Here's how the part is built. I have some questions about the finished solid (model axes, mm). Coordinates: 2 decimals unless noted, no trailing zeros. Write each loop counter-clockwise with the first axis right and the second up, starting at its lowest first coordinate (ties: lowest second). Pieces come first, ordered by that corner, then holes.
Item 1: If we section it at C-C (z = 3.4): Count the separate pieces of the cut face and the enclosed holes in it, then the cut area to 3 significant figures.
Item 2: If we section it at B-B (x = 390.5): Please give me the cut outline in (y, z).
Item 3: If I drill on line 1 (X direction, y = 30, z = 3.5); line 2 (Y direction, x = 30, z = 2.1); line 3 (Y direction, x = 403, z = 1.2), over which ranges is the centre line in solid material (lowest first)?
Item 4: If we section it at A-A (x = 97.5): Please give me the cut outline in (y, z), then the cut area to 3 significant figures.
from build123d import *

# Parameters (mm, degrees)
BOSS_EXTRU_1_DEPTH         = 5
D_GAGEMENT_M51_D           = 5.5
D_GAGEMENT_M51_CSINK_D     = 5.55
D_GAGEMENT_M51_CSINK_ANGLE = 90
ENL_V_MAT_EXTRU_1_DEPTH    = 560.039354608
D_GAGEMENT_M52_D           = 5.5
D_GAGEMENT_M52_CSINK_D     = 6
D_GAGEMENT_M52_CSINK_ANGLE = 90
ENL_V_MAT_EXTRU_2_DEPTH    = 560.039354608
ENL_V_MAT_EXTRU_3_DEPTH    = 560.039354608
ESQUISSE15_R               = 2.5
ENL_V_MAT_EXTRU_4_DEPTH    = 560.039354608


with BuildPart() as part:
    # Esquisse1 → Boss.-Extru.1 (new body)
    with BuildSketch(Plane.XY):
        with BuildLine():
            Line((30, 0), (470, 0))
            ThreePointArc((470, 0), (491.213203436, 8.786796564), (500, 30))
            Line((500, 30), (500, 220))
            ThreePointArc((500, 220), (491.213203436, 241.213203436), (470, 250))
            Line((470, 250), (30, 250))
            ThreePointArc((30, 250), (8.786796564, 241.213203436), (0, 220))
            Line((0, 220), (0, 30))
            ThreePointArc((0, 30), (8.786796564, 8.786796564), (30, 0))
        make_face()
    extrude(amount=BOSS_EXTRU_1_DEPTH)

    # Dégagement M51 (through all)
    with Locations(Plane(origin=(0, 0, 0), x_dir=(-1, 0, 0), z_dir=(0, 0, -1))):
        with Locations((-470, 220), (-470, 30), (-30, 30), (-30, 220)):
            CounterSinkHole(D_GAGEMENT_M51_D / 2, D_GAGEMENT_M51_CSINK_D / 2, counter_sink_angle=D_GAGEMENT_M51_CSINK_ANGLE)

    # Esquisse8 → Enlèv. mat.-Extru.1 (cut, through all)
    with BuildSketch(Plane.XY.offset(5)):
        with BuildLine():
            Line((72, 225), (152, 225))
            ThreePointArc((152, 225), (153.414213562, 224.414213562), (154, 223))
            Line((154, 223), (154, 215))
            ThreePointArc((154, 215), (153.414213562, 213.585786438), (152, 213))
            Line((152, 213), (72, 213))
            ThreePointArc((72, 213), (70.585786438, 213.585786438), (70, 215))
            Line((70, 215), (70, 223))
            ThreePointArc((70, 223), (70.585786438, 224.414213562), (72, 225))
        make_face()
        with BuildLine():
            Line((346, 223), (346, 215))
            ThreePointArc((346, 215), (346.585786438, 213.585786438), (348, 213))
            Line((348, 213), (428, 213))
            ThreePointArc((428, 213), (429.414213562, 213.585786438), (430, 215))
            Line((430, 215), (430, 223))
            ThreePointArc((430, 223), (429.414213562, 224.414213562), (428, 225))
            Line((428, 225), (348, 225))
            ThreePointArc((348, 225), (346.585786438, 224.414213562), (346, 223))
        make_face()
    extrude(amount=-ENL_V_MAT_EXTRU_1_DEPTH, mode=Mode.SUBTRACT)

    # Dégagement M52 (through all)
    with Locations(Plane.XY.offset(5)):
        with Locations((60, 238), (440, 238), (250, 238)):
            CounterSinkHole(D_GAGEMENT_M52_D / 2, D_GAGEMENT_M52_CSINK_D / 2, counter_sink_angle=D_GAGEMENT_M52_CSINK_ANGLE)

    # Esquisse13 → Enlèv. mat.-Extru.2 (cut, through all)
    with BuildSketch(Plane(origin=(0, 0, 0), x_dir=(-1, 0, 0), z_dir=(0, 0, -1))):
        with BuildLine():
            Line((-105, 88), (-105, 62))
            ThreePointArc((-105, 62), (-104.414213562, 60.585786438), (-103, 60))
            Line((-103, 60), (-82, 60))
            ThreePointArc((-82, 60), (-80.585786438, 60.585786438), (-80, 62))
            Line((-80, 62), (-80, 88))
            ThreePointArc((-80, 88), (-80.585786438, 89.414213562), (-82, 90))
            Line((-82, 90), (-103, 90))
            ThreePointArc((-103, 90), (-104.414213562, 89.414213562), (-105, 88))
        make_face()
    extrude(amount=-ENL_V_MAT_EXTRU_2_DEPTH, mode=Mode.SUBTRACT)

    # Esquisse14 → Enlèv. mat.-Extru.3 (cut, through all)
    with BuildSketch(Plane.XY.offset(5)):
        with BuildLine():
            Line((144.742586668, 75), (148.952586668, 75))
            ThreePointArc((148.952586668, 75), (146.847586668, 79.179927883), (144.742586668, 75))
        make_face()
    extrude(amount=-ENL_V_MAT_EXTRU_3_DEPTH, mode=Mode.SUBTRACT)

    # Esquisse15 → Enlèv. mat.-Extru.4 (cut, through all)
    with BuildSketch(Plane.XY.offset(5)):
        with Locations((164.292422871, 76.559927883)):
            Circle(ESQUISSE15_R)
    extrude(amount=-ENL_V_MAT_EXTRU_4_DEPTH, mode=Mode.SUBTRACT)


solid = part.part
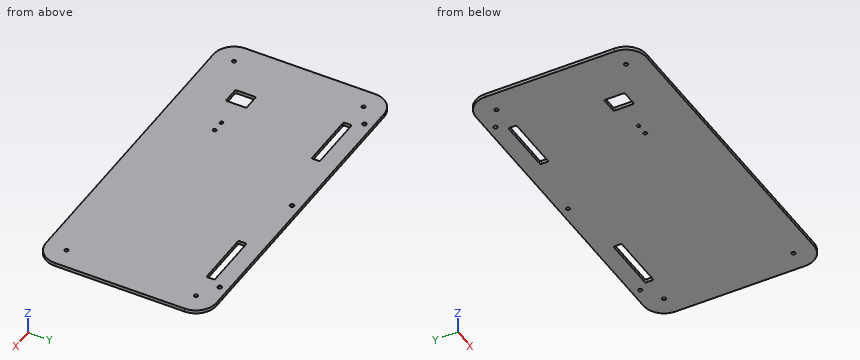
Answer list:
1. separate pieces: 1
1. enclosed holes: 12
1. area: 121,000 mm2
2. outline: (0, 0) - (213, 0) - (213, 5) - (0, 5) - close; (225, 0) - (250, 0) - (250, 5) - (225, 5) - close
3. line 1: x = 0 to 27.25, 32.75 to 467.25, 472.75 to 500
3. line 2: y = 0 to 27.25, 32.75 to 217.25, 222.75 to 250
3. line 3: y = 0 to 213, 225 to 250
4. outline: (0, 0) - (60, 0) - (60, 5) - (0, 5) - close; (90, 0) - (213, 0) - (213, 5) - (90, 5) - close; (225, 0) - (250, 0) - (250, 5) - (225, 5) - close
4. area: 1,040 mm2
